Check sheet for the drawn part. Datum: minimum x, y, z corner. Units: mm. A direction names the side the tool comes from. Round coordinates to 2 decimals unless told otherwise and drop trailing zeros. Order: outer loops, then holes, each group sorted by start corner. A loop starts at its lowest first (then second) coordinate and runs counter-clockwise, first axis right, second up. Notation, with made-up numbers: M 3.25,-34 L 36.25,-34 A16 cw 36.25,-9 Z; hole C 4,51.25 d10. An arc over 180 degrees is marked long. Use one line per item in the form item = value. Start each with the question number.
Item 1: Cross-section at B-B on x = 4.3. Enter the section's corners in (y, z), then the cut area to 3 significant figures.
Item 2: Release check for a two-part mould opening along Y. For the marked faces 3, 4 and 5 record: +Y half, -Y half, draft (parallel to the pull), parting line (faces both ways), or undercut.
Item 3: Cross-section at A-A on z = 11. Enter the section's corners in (x, y), then the cut area to 3 significant figures.
Item 4: Tool access check on the marked faces 1 and 2. Record the directions out of +Z, -Z, +X, -X, +Y, -Y that give a thin tool (end or side, any length) a straight path to the whole face; none if there is none.
Item 5: Thickness scan on probe 1 along Z at (x, y) = (1.85, 11); probe 2 along Y at (x, z) = (1.45, 11); probe 3 along Z at (x, y) = (0.5, 16) (3 decimals). Record the ranges inside material, lowest first. Write a range as [from, to].
Item 6: Cross-section at C-C on y = 8.5. Enter the section's corners in (x, z).
Item 7: Go/stop test with a flat-tipped pin: pin 1 Ø6 at (y, z) = (16.5, 10.5) entering from +X. Record where the tip stops, or that it passes through.
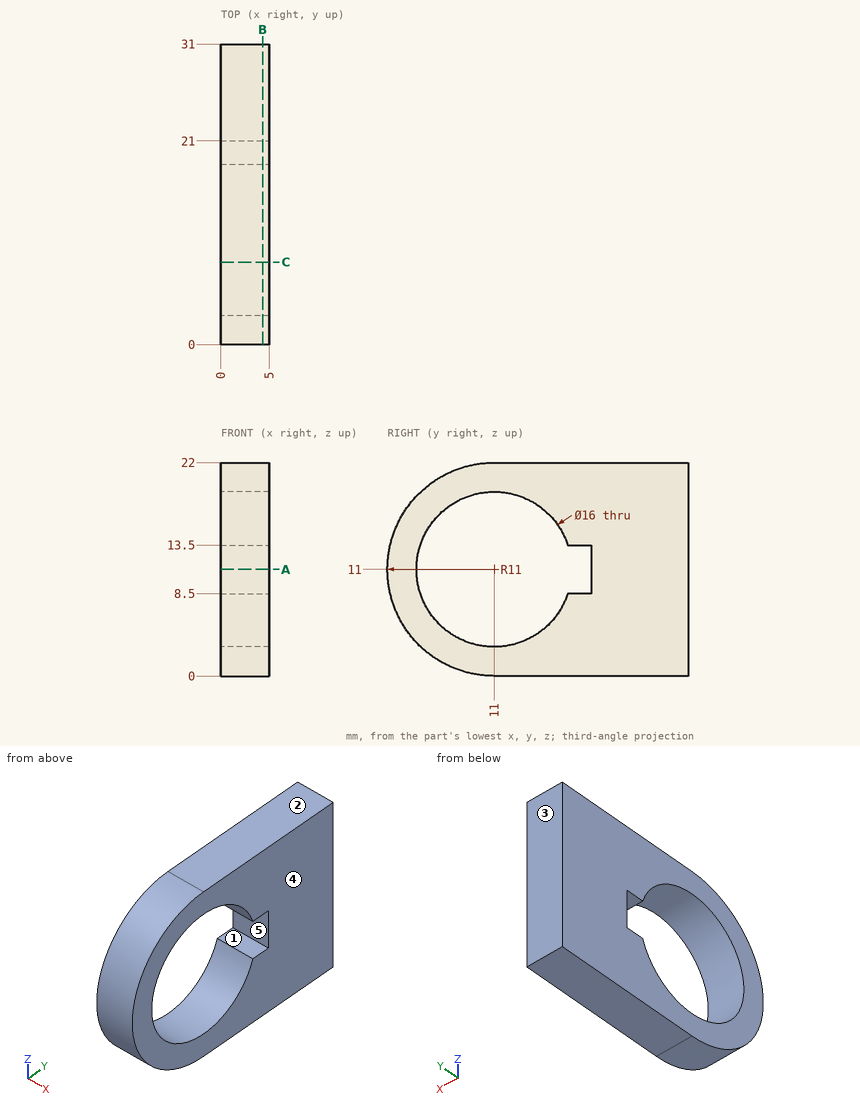
Output values:
q1.outline = M 11,0 L 31,0 L 31,22 L 11,22 A11 ccw Z; hole M 18.6,8.5 L 21,8.5 L 21,13.5 L 18.6,13.5 A8 ccw long Z
q1.area = 418 mm2
q2.face_3 = +Y half
q2.face_4 = draft
q2.face_5 = undercut
q3.outline = M 0,0 L 5,0 L 5,3 L 0,3 Z; M 0,21 L 5,21 L 5,31 L 0,31 Z
q3.area = 65.0 mm2
q4.face_1 = +X, -X
q4.face_2 = +Z, +X, -X, +Y, -Y
q5.probe_1 = [0, 3], [19, 22]
q5.probe_2 = [0, 3], [21, 31]
q5.probe_3 = [0, 4.755], [17.245, 22]
q6.outline = M 0,0.29 L 5,0.29 L 5,3.4 L 0,3.4 Z; M 0,18.6 L 5,18.6 L 5,21.71 L 0,21.71 Z
q7.pin_1 = 5
